from build123d import *

# Parameters (mm, degrees)
BOSS_EXTRUDE1_DEPTH     = 420
SKETCH2_R               = 3
CUT_EXTRUDE1_DEPTH      = 4.5
SKETCH3_R               = 1.75
CUT_EXTRUDE2_DEPTH      = 421.066958948
LPATTERN1_COUNT         = 4
LPATTERN1_PITCH         = 25
MIRROR1_COPY_1_SKETCH_R = 3
MIRROR1_COPY_1_DEPTH    = 4.5
MIRROR1_COPY_2_SKETCH_R = 3
MIRROR1_COPY_2_DEPTH    = 4.5
MIRROR1_COPY_3_SKETCH_R = 3
MIRROR1_COPY_3_DEPTH    = 4.5
MIRROR1_COPY_4_SKETCH_R = 1.75
MIRROR1_COPY_4_DEPTH    = 421.066958948
MIRROR1_COPY_5_SKETCH_R = 1.75
MIRROR1_COPY_5_DEPTH    = 421.066958948
MIRROR1_COPY_6_SKETCH_R = 1.75
MIRROR1_COPY_6_DEPTH    = 421.066958948
SKETCH5_R               = 3
SKETCH5_W               = 0.5
SKETCH5_H               = 35
CUT_EXTRUDE3_DEPTH      = 421.119030752


with BuildPart() as part:
    # Sketch1 → Boss-Extrude1 (new body)
    with BuildSketch(Plane.XY):
        with BuildLine():
            Line((6, -3.5), (6, 0.368911094))
            ThreePointArc((6, 0.368911094), (5.63354293, 0.61854293), (5.383911094, 0.985))
            Line((5.383911094, 0.985), (4.92112495, 0.985))
            ThreePointArc((4.92112495, 0.985), (4.265, 1.46), (4.92112495, 1.935))
            Line((4.92112495, 1.935), (5.383911094, 1.935))
            ThreePointArc((5.383911094, 1.935), (5.63354293, 2.30145707), (6, 2.551088906))
            Line((6, 2.551088906), (6, 3.5))
            Line((6, 3.5), (5.5, 4))
            Line((5.5, 4), (-5.5, 4))
            Line((-5.5, 4), (-6, 3.5))
            Line((-6, 3.5), (-6, 2.551088906))
            ThreePointArc((-6, 2.551088906), (-5.63354293, 2.30145707), (-5.383911094, 1.935))
            Line((-5.383911094, 1.935), (-4.92112495, 1.935))
            ThreePointArc((-4.92112495, 1.935), (-4.265, 1.46), (-4.92112495, 0.985))
            Line((-4.92112495, 0.985), (-5.383911094, 0.985))
            ThreePointArc((-5.383911094, 0.985), (-5.63354293, 0.61854293), (-6, 0.368911094))
            Line((-6, 0.368911094), (-6, -3.5))
            Line((-6, -3.5), (-5.5, -4))
            Line((-5.5, -4), (5.5, -4))
            Line((5.5, -4), (6, -3.5))
        make_face()
    extrude(amount=BOSS_EXTRUDE1_DEPTH)

    # Sketch2 → Cut-Extrude1 (cut)
    with BuildSketch(Plane(origin=(0, 4, 0), x_dir=(1, 0, 0), z_dir=(0, 1, 0))):
        with Locations(Location((0, -12.5, 0), (0, 0, 180))):
            Circle(SKETCH2_R)
    cut_extrude1 = extrude(amount=-CUT_EXTRUDE1_DEPTH, mode=Mode.SUBTRACT)

    # Sketch3 → Cut-Extrude2 (cut, through all)
    with BuildSketch(Plane(origin=(0, -0.5, 0), x_dir=(1, 0, 0), z_dir=(0, 1, 0))):
        with Locations(Location((0, -12.5, 0), (0, 0, 180))):
            Circle(SKETCH3_R)
    cut_extrude2 = extrude(amount=-CUT_EXTRUDE2_DEPTH, mode=Mode.SUBTRACT)

    # LPattern1: Cut-Extrude1, Cut-Extrude2 ×4
    with Locations(*[(0, 0, i * LPATTERN1_PITCH) for i in range(1, LPATTERN1_COUNT)]):
        add(cut_extrude1, mode=Mode.SUBTRACT)
        add(cut_extrude2, mode=Mode.SUBTRACT)

    # Mirror1: Cut-Extrude1, Cut-Extrude2 across plane
    add(cut_extrude1.mirror(Plane.XY.offset(210)), mode=Mode.SUBTRACT)
    add(cut_extrude2.mirror(Plane.XY.offset(210)), mode=Mode.SUBTRACT)

    # Mirror1 copy 1 sketch → Mirror1 copy 1 (cut)
    with BuildSketch(Plane(origin=(0, 4, 395), x_dir=(1, 0, 0), z_dir=(0, 1, 0))):
        with Locations((0, 12.5)):
            Circle(MIRROR1_COPY_1_SKETCH_R)
    extrude(amount=-MIRROR1_COPY_1_DEPTH, mode=Mode.SUBTRACT)

    # Mirror1 copy 2 sketch → Mirror1 copy 2 (cut)
    with BuildSketch(Plane(origin=(0, 4, 370), x_dir=(1, 0, 0), z_dir=(0, 1, 0))):
        with Locations((0, 12.5)):
            Circle(MIRROR1_COPY_2_SKETCH_R)
    extrude(amount=-MIRROR1_COPY_2_DEPTH, mode=Mode.SUBTRACT)

    # Mirror1 copy 3 sketch → Mirror1 copy 3 (cut)
    with BuildSketch(Plane(origin=(0, 4, 345), x_dir=(1, 0, 0), z_dir=(0, 1, 0))):
        with Locations((0, 12.5)):
            Circle(MIRROR1_COPY_3_SKETCH_R)
    extrude(amount=-MIRROR1_COPY_3_DEPTH, mode=Mode.SUBTRACT)

    # Mirror1 copy 4 sketch → Mirror1 copy 4 (cut, through all)
    with BuildSketch(Plane(origin=(0, -0.5, 395), x_dir=(1, 0, 0), z_dir=(0, 1, 0))):
        with Locations((0, 12.5)):
            Circle(MIRROR1_COPY_4_SKETCH_R)
    extrude(amount=-MIRROR1_COPY_4_DEPTH, mode=Mode.SUBTRACT)

    # Mirror1 copy 5 sketch → Mirror1 copy 5 (cut, through all)
    with BuildSketch(Plane(origin=(0, -0.5, 370), x_dir=(1, 0, 0), z_dir=(0, 1, 0))):
        with Locations((0, 12.5)):
            Circle(MIRROR1_COPY_5_SKETCH_R)
    extrude(amount=-MIRROR1_COPY_5_DEPTH, mode=Mode.SUBTRACT)

    # Mirror1 copy 6 sketch → Mirror1 copy 6 (cut, through all)
    with BuildSketch(Plane(origin=(0, -0.5, 345), x_dir=(1, 0, 0), z_dir=(0, 1, 0))):
        with Locations((0, 12.5)):
            Circle(MIRROR1_COPY_6_SKETCH_R)
    extrude(amount=-MIRROR1_COPY_6_DEPTH, mode=Mode.SUBTRACT)

    # Sketch5 → Cut-Extrude3 (cut, through all)
    # profile 1 of 8: a face of its own
    with BuildSketch(Plane(origin=(0, 4, 0), x_dir=(1, 0, 0), z_dir=(0, 1, 0))):
        with BuildLine():
            Line((-1.658312395, -385), (-5.5, -385))
            Line((-5.5, -385), (-5.5, -420))
            Line((-5.5, -420), (5.5, -420))
            Line((5.5, -420), (5.5, -385))
            Line((5.5, -385), (1.658312395, -385))
            ThreePointArc((1.658312395, -385), (0, -385.5), (-1.658312395, -385))
        make_face()
        with Locations((0, -407.5)):
            Circle(SKETCH5_R, mode=Mode.SUBTRACT)
    # profile 2 of 8: a face of its own
    with BuildSketch(Plane(origin=(0, 4, 0), x_dir=(1, 0, 0), z_dir=(0, 1, 0))):
        with Locations((-5.75, -402.5)):
            Rectangle(SKETCH5_W, SKETCH5_H)
    # profile 3 of 8: a face of its own
    with BuildSketch(Plane(origin=(0, 4, 0), x_dir=(1, 0, 0), z_dir=(0, 1, 0))):
        with Locations((5.75, -402.5)):
            Rectangle(SKETCH5_W, SKETCH5_H)
    # profile 4 of 8: a face of its own
    with BuildSketch(Plane(origin=(0, 4, 0), x_dir=(1, 0, 0), z_dir=(0, 1, 0))):
        with Locations((0, -407.5)):
            Circle(SKETCH5_R)
    # profile 5 of 8: a face of its own
    with BuildSketch(Plane(origin=(0, 4, 0), x_dir=(1, 0, 0), z_dir=(0, 1, 0))):
        with BuildLine():
            Line((-5.5, 0), (-5.5, -35))
            Line((-5.5, -35), (-1.658312395, -35))
            ThreePointArc((-1.658312395, -35), (0, -34.5), (1.658312395, -35))
            Line((1.658312395, -35), (5.5, -35))
            Line((5.5, -35), (5.5, 0))
            Line((5.5, 0), (-5.5, 0))
        make_face()
        with Locations((0, -12.5)):
            Circle(SKETCH5_R, mode=Mode.SUBTRACT)
    # profile 6 of 8: a face of its own
    with BuildSketch(Plane(origin=(0, 4, 0), x_dir=(1, 0, 0), z_dir=(0, 1, 0))):
        with Locations((0, -12.5)):
            Circle(SKETCH5_R)
    # profile 7 of 8: a face of its own
    with BuildSketch(Plane(origin=(0, 4, 0), x_dir=(1, 0, 0), z_dir=(0, 1, 0))):
        with Locations((5.75, -17.5)):
            Rectangle(SKETCH5_W, SKETCH5_H)
    # profile 8 of 8: a face of its own
    with BuildSketch(Plane(origin=(0, 4, 0), x_dir=(1, 0, 0), z_dir=(0, 1, 0))):
        with Locations((-5.75, -17.5)):
            Rectangle(SKETCH5_W, SKETCH5_H)
    extrude(amount=-CUT_EXTRUDE3_DEPTH, mode=Mode.SUBTRACT)


solid = part.part
Could you check a few things on this model? Use its own coordinates, in mm. A direction names the side the tool comes from. Give positions to 0.01 mm unless a question says otherwise; leave off trailing zeros. Write each loop counter-clockwise with the first axis right and the second up, starting at its lowest first coordinate (ties: lowest second). Pieces come first, ordered by that corner, then holes. Notation, with made-up numbers: (25.5, 87) -> (65.5, 87) arc R22 cw to (65.5, 113) -> close; hole circle Ø8 at (77, 11.5). An arc over 180 degrees is marked (long way). Answer as a JSON object with one key per item and string values.
Q1. We'd pull the mould along X, two halves only. Please class faces 1 (the cylindrical face through (0.1, 1.8, 379.5)), 2 (the flat face through (0, -4, 208)): released by +X, released by -X, zero draft, split by the parting line, or undercut.
Taken from the geometry:
{"face 1": "undercut", "face 2": "zero draft"}
Q2. Please list where these lines run through material, in increasing order: L1, parallel to Z at x = 0, y = 1.25; L2, parallel to Y at x = -4.5, z = 102.5; L3, parallel to Z at x = 2.5, y = -3.5.
Taken from the geometry:
{"L1": "z = 40.5 to 59.5, 65.5 to 84.5, 90.5 to 329.5, 335.5 to 354.5, 360.5 to 379.5", "L2": "y = -4 to 1.04, 1.88 to 4", "L3": "z = 35 to 385"}
Q3. Suppose I cut it at A-A on z = 233. Write out the boundary of the cut face in (x, y) (3 decimals).
Taken from the geometry:
{"outline": "(-6, -3.5) -> (-5.5, -4) -> (5.5, -4) -> (6, -3.5) -> (6, 0.369) arc R1.19 cw to (5.384, 0.985) -> (4.921, 0.985) arc R0.5 cw (long way) to (4.921, 1.935) -> (5.384, 1.935) arc R1.19 cw to (6, 2.551) -> (6, 3.5) -> (5.5, 4) -> (-5.5, 4) -> (-6, 3.5) -> (-6, 2.551) arc R1.19 cw to (-5.384, 1.935) -> (-4.921, 1.935) arc R0.5 cw (long way) to (-4.921, 0.985) -> (-5.384, 0.985) arc R1.19 cw to (-6, 0.369) -> close"}
Q4. Which directions (+Z, -Z, +X, -X, +Y, -Y) give clear straight access to the entire face, cutting with the end or side of a thin tool? Please do faces 3 (the cylindrical face through (-0.1, 1.8, 40.5)), 4 (the flat face through (0, 4, 208)).
Taken from the geometry:
{"face 3": "+Y", "face 4": "+Z, -Z, +X, -X, +Y"}
Q5. Will these pins go through, and if not, where does the flat tip stop? pin 1 Ø1.3 at (x, y) = (-3.5, 0) entering from +Z; pin 2 Ø2 at (x, y) = (4, -0.5) entering from -Z; pin 3 Ø1.8 at (x, z) = (1, 36) entering from +Y.
Taken from the geometry:
{"pin 1": "stops at z = 385", "pin 2": "stops at z = 35", "pin 3": "stops at y = -0.5"}
